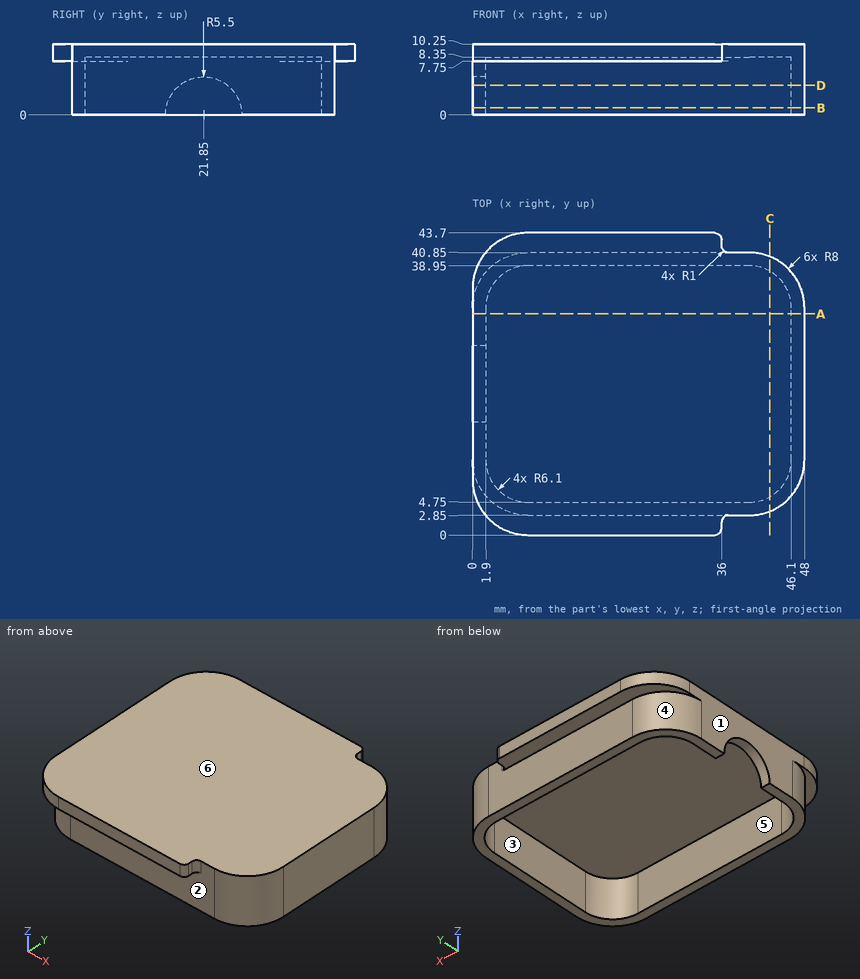
The figure shows three views and two pictorial views of one solid part (mm, origin at its lowest corner). Answer the questions. A direction names the side the tool comes from. Round coordinates to 2 decimals unless told otherwise and drop trailing zeros. Write each loop counter-clockwise with the first axis right and the second up, starting at its lowest first coordinate (ties: lowest second). Pieces come first, ordered by that corner, then holes. Notation, with made-up numbers: (-7.5, 43) -> (51.5, 43) arc R25 cw to (51.5, 75) -> close; hole circle Ø11 at (-14.75, -27.5). An arc over 180 degrees is marked (long way). Answer as a JSON object with one key per item and string values. Group by question number.
Q1. Section A-A (y = 32) is taken. Write down the section's boundary in (x, z), plus the area to 3 significant figures.
Q2. Section B-B (z = 1) is taken. Write down the section's boundary in (x, y), plus the area to 3 significant figures.
Q3. Section D-D (z = 4.25) is taken. Write down the section's boundary in (x, y), plus the area to 3 significant figures.
Q4. Which of the six approach directions +Z, -Z, +X, -X, +Y, -Y give full straight-line access (tool end or side, diameter ignored) to the marked faces 4, 5 and 6?
Q5. Determine the mould class of the marked faces 1, 2 and 3 for opening direction X: pulls with the +X half, pulls with the -X half, needs draft (parallel to the pull), parting line crosses it, or undercut.
Q6. Straight lines are drawn through the part: line 1 along X through (y, z) = (28.5, 6.5); line 2 along Y through (x, z) = (39.5, 1.75); line 3 along Z through (x, y) = (42.5, 37.5). For each, find the intervals that lie inside material, in ascending order.
Q7. Each of these flat-tipped pins is pushed along its axis until it touches: pin 1 Ø0.9 at (y, z) = (1.5, 9.5) entering from +X (3 decimals); pin 2 Ø2 at (y, z) = (21, 2.5) entering from -X; pin 3 Ø4 at (x, y) = (12, 17) entering from -Z. Where does it stop, or does it pass through?
Q8. Section C-C (x = 43) is taken. Write down the section's boundary in (y, z), plus the area to 3 significant figures.
Check values:
{
 "1": {"outline": "(0, 0) -> (1.9, 0) -> (1.9, 8.35) -> (46.1, 8.35) -> (46.1, 0) -> (48, 0) -> (48, 10.25) -> (0, 10.25) -> close", "area": "123 mm^2"},
 "2": {"outline": "(0, 10.85) arc R8 ccw to (8, 2.85) -> (40, 2.85) arc R8 ccw to (48, 10.85) -> (48, 32.85) arc R8 ccw to (40, 40.85) -> (8, 40.85) arc R8 ccw to (0, 32.85) -> (0, 27.26) -> (1.9, 27.26) -> (1.9, 32.85) arc R6.1 cw to (8, 38.95) -> (40, 38.95) arc R6.1 cw to (46.1, 32.85) -> (46.1, 10.85) arc R6.1 cw to (40, 4.75) -> (8, 4.75) arc R6.1 cw to (1.9, 10.85) -> (1.9, 16.44) -> (0, 16.44) -> close", "area": "269 mm^2"},
 "3": {"outline": "(0, 10.85) arc R8 ccw to (8, 2.85) -> (40, 2.85) arc R8 ccw to (48, 10.85) -> (48, 32.85) arc R8 ccw to (40, 40.85) -> (8, 40.85) arc R8 ccw to (0, 32.85) -> (0, 25.34) -> (1.9, 25.34) -> (1.9, 32.85) arc R6.1 cw to (8, 38.95) -> (40, 38.95) arc R6.1 cw to (46.1, 32.85) -> (46.1, 10.85) arc R6.1 cw to (40, 4.75) -> (8, 4.75) arc R6.1 cw to (1.9, 10.85) -> (1.9, 18.36) -> (0, 18.36) -> close", "area": "276 mm^2"},
 "4": {"face 4": "-Z, -X, +Y", "face 5": "-Z", "face 6": "+Z, +X, -X, +Y, -Y"},
 "5": {"face 1": "pulls with the -X half", "face 2": "needs draft", "face 3": "undercut"},
 "6": {"line 1": "0 to 1.9, 46.1 to 48", "line 2": "2.85 to 4.75, 38.95 to 40.85", "line 3": "8.35 to 10.25"},
 "7": {"pin 1": "x = 36.005", "pin 2": "x = 46.1", "pin 3": "z = 8.35"},
 "8": {"outline": "(3.43, 0) -> (5.54, 0) -> (5.54, 8.35) -> (38.16, 8.35) -> (38.16, 0) -> (40.27, 0) -> (40.27, 10.25) -> (3.43, 10.25) -> close", "area": "105 mm^2"}
}
